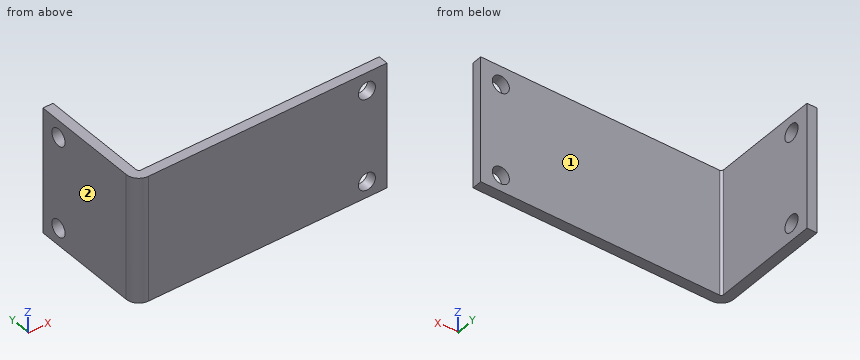
```python
from build123d import *

# Parameters (mm, degrees)
SM_BASE_FLANGE_1_DEPTH = 25
SKETCH_6_R             = 1.7
CUT_EXTRUDE_1_DEPTH    = 10
SKETCH_7_R             = 1.7
CUT_EXTRUDE_2_DEPTH    = 10


# Sheet-metal steps are written as plain solids
with BuildPart() as part:
    # Sketch 1 → 基体-法兰1 (new body)
    with BuildSketch(Plane.XY):
        with BuildLine():
            Line((0, 24), (0, 2.5))
            ThreePointArc((0, 2.5), (0.732233047, 0.732233047), (2.5, 0))
            Line((2.5, 0), (50, 0))
            Line((50, 0), (50, 2))
            Line((50, 2), (2.5, 2))
            ThreePointArc((2.5, 2), (2.146446609, 2.146446609), (2, 2.5))
            Line((2, 2.5), (2, 24))
            Line((2, 24), (0, 24))
        make_face()
    extrude(amount=SM_BASE_FLANGE_1_DEPTH)

    # 草图6 → 切除-拉伸1 (cut)
    with BuildSketch(Plane(origin=(2, 0, 0), x_dir=(0, 0, -1), z_dir=(1, 0, 0))):
        with Locations((-3.4, 20)):
            Circle(SKETCH_6_R)
        with Locations((-21.6, 20)):
            Circle(SKETCH_6_R)
    extrude(amount=-CUT_EXTRUDE_1_DEPTH, mode=Mode.SUBTRACT)

    # 草图7 → 切除-拉伸2 (cut)
    with BuildSketch(Plane(origin=(0, 2, 0), x_dir=(1, 0, 0), z_dir=(0, 1, 0))):
        with Locations(Location((46, -3.184253604, 0), (0, 0, 270))):
            Circle(SKETCH_7_R)
        with Locations(Location((46, -21.384253604, 0), (0, 0, 270))):
            Circle(SKETCH_7_R)
    extrude(amount=-CUT_EXTRUDE_2_DEPTH, mode=Mode.SUBTRACT)


solid = part.part
```
Read the model definition and answer for the solid it produces. Units are mm, in the model's axes. Face numbers are marked on the shaded views. A direction names the side the tool comes from. Coordinates: 2 decimals unless noted, no trailing zeros. Loops run counter-clockwise (first coordinate to the right, second up) from the corner with the lowest first, then second, coordinate; pieces in that order, holes last.
(1) Consider line 1 along Y through (x, z) = (6.5, 2.75); line 2 along Y through (x, z) = (0.95, 3.4). Determine where each line is inside the solid, lowest interval first.
Solution:
line 1: y = 0 to 2
line 2: y = 0.54 to 18.3, 21.7 to 24
(2) A tool of negligible diameter and unlimited length cuts with its end or side. For the marked faces 1 and 2, from which of +Z, -Z, +X, -X, +Y, -Y can it reach the whole face along a straight path? Write none if from no direction.
Solution:
face 1: +Z, -Z, +X, +Y
face 2: +Z, -Z, -X, +Y, -Y
(3) The part is cut by section A-A (x = 46). Determine the outline of the cut face in (y, z).
Solution:
outline: (0, 0) - (2, 0) - (2, 1.48) - (0, 1.48) - close; (0, 4.88) - (2, 4.88) - (2, 19.68) - (0, 19.68) - close; (0, 23.08) - (2, 23.08) - (2, 25) - (0, 25) - close
(4) Flat-ended cylindrical pins translate along their axes: pin 1 Ø1.5 at (x, z) = (11, 13.5) entering from -Y; pin 2 Ø6 at (x, z) = (23, 20.5) entering from +Y; pin 3 Ø4 at (y, z) = (20, 21.6) entering from +X. Find the tip coordinate at first contact, or state that the pin passes through.
Solution:
pin 1: stops at y = 0
pin 2: stops at y = 2
pin 3: stops at x = 2
(5) The part is cut by section C-C (z = 4.25). Determine the outline of the cut face in (x, y), and give its area (3 significant figures).
Solution:
outline: (0, 2.5) arc R2.5 ccw to (2.5, 0) - (44.68, 0) - (44.68, 2) - (2.5, 2) arc R0.5 cw to (2, 2.5) - (2, 18.53) - (0, 18.53) - close; (0, 21.47) - (2, 21.47) - (2, 24) - (0, 24) - close; (47.32, 0) - (50, 0) - (50, 2) - (47.32, 2) - close
area: 132 mm2
(6) The part is cut by section D-D (z = 6.75). Determine the outline of the cut face in (x, y), and give its area (3 significant figures).
Solution:
outline: (0, 2.5) arc R2.5 ccw to (2.5, 0) - (50, 0) - (50, 2) - (2.5, 2) arc R0.5 cw to (2, 2.5) - (2, 24) - (0, 24) - close
area: 143 mm2
(7) The part is cut by section B-B (y = 20). Determine the outline of the cut face in (x, z).
Solution:
outline: (0, 0) - (2, 0) - (2, 1.7) - (0, 1.7) - close; (0, 5.1) - (2, 5.1) - (2, 19.9) - (0, 19.9) - close; (0, 23.3) - (2, 23.3) - (2, 25) - (0, 25) - close
